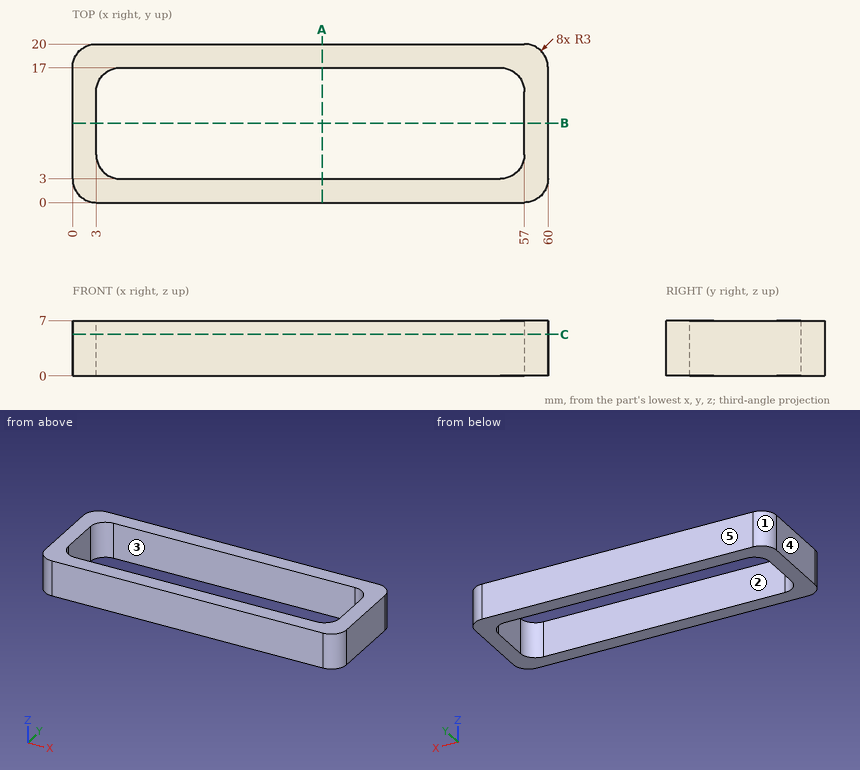
Could you check a few things on this drawing? It's one solid part, dimensions in mm from its lowest x, y, z. A direction names the side the tool comes from. Coordinates: 2 decimals unless noted, no trailing zeros. Order: outer loops, then holes, each group sorted by start corner. A loop starts at its lowest first (then second) coordinate and runs counter-clockwise, first axis right, second up. Notation, with made-up numbers: (51, 81) -> (75, 81) arc R11 ccw to (75, 100) -> close; hole circle Ø5 at (50, 12). An arc over 180 degrees is marked (long way). Answer in a Markdown table with one row per item.
(1) Thinking about a two-plate mould opening in Y: for the marked faces 3, 4 and 5, which applies, +Y half, -Y half, draft (parallel to the pull), parting line (faces both ways), or undercut?
Answer key:
| item | result |
|---|---|
| face 3 | undercut |
| face 4 | draft |
| face 5 | +Y half |
(2) Please list where these lines run through material, in increasing order: probe 1 along X at (y, z) = (11, 6); probe 2 along Y at (x, z) = (36, 1.25); probe 3 along X at (y, z) = (16.25, 1).
Answer key:
| item | result |
|---|---|
| probe 1 | 0 to 3, 57 to 60 |
| probe 2 | 0 to 3, 17 to 20 |
| probe 3 | 0 to 4.02, 55.98 to 60 |
(3) I want a section at B-B on y = 10. List the corners of the cut face in (x, z) for me, then the cut area to 3 significant figures.
Answer key:
| item | result |
|---|---|
| outline | (0, 0) -> (3, 0) -> (3, 7) -> (0, 7) -> close; (57, 0) -> (60, 0) -> (60, 7) -> (57, 7) -> close |
| area | 42.0 mm^2 |
(4) I want a section at C-C on z = 5.25. List the corners of the cut face in (x, y) for me.
Answer key:
| item | result |
|---|---|
| outline | (0, 3) arc R3 ccw to (3, 0) -> (57, 0) arc R3 ccw to (60, 3) -> (60, 17) arc R3 ccw to (57, 20) -> (3, 20) arc R3 ccw to (0, 17) -> close; hole (3, 6) arc R3 ccw to (6, 3) -> (54, 3) arc R3 ccw to (57, 6) -> (57, 14) arc R3 ccw to (54, 17) -> (6, 17) arc R3 ccw to (3, 14) -> close |
(5) On a 3-axis mill with a long thin cutter (end or side, diameter ignored), from which of +Z, -Z, +X, -X, +Y, -Y can I reach the whole of each face in a straight line? I mean the marked faces 1 and 2. Say none if no direction works.
Answer key:
| item | result |
|---|---|
| face 1 | +Z, -Z, -X, +Y |
| face 2 | +Z, -Z |
(6) Will this pin go through, and if not, where does the flat tip stop? pin 1 Ø6 at (x, y) = (10, 13) entering from -Z.
Answer key:
| item | result |
|---|---|
| pin 1 | through |
(7) I want a section at A-A on x = 31.5. List the corners of the cut face in (y, z) for me, then the cut area to 3 significant figures.
Answer key:
| item | result |
|---|---|
| outline | (0, 0) -> (3, 0) -> (3, 7) -> (0, 7) -> close; (17, 0) -> (20, 0) -> (20, 7) -> (17, 7) -> close |
| area | 42.0 mm^2 |
